Autodesk Inventor part; units mm, degrees
ref_plane "YZ Plane" through (0, 0, 0) normal (1, 0, 0) x (0, 1, 0)
ref_plane "XZ Plane" through (0, 0, 0) normal (0, 1, 0) x (-1, 0, 0)
ref_plane "XY Plane" through (0, 0, 0) normal (0, 0, 1) x (1, 0, 0)
sketch "Sketch1" plane through (0, 0, 0) normal (0, 1, 0) x (-1, 0, 0)
  line L0 (-4, 0) -> (-2, 3.4641)
  line L1 (-2, 3.4641) -> (2, 3.4641)
  line L2 (2, 3.4641) -> (4, 0)
  line L3 (4, 0) -> (2, -3.4641)
  line L4 (2, -3.4641) -> (-2, -3.4641)
  line L5 (-2, -3.4641) -> (-4, 0)
  point P0 (0, 0)
  point P1 (0, 0)
  dimension "d1" = 8
extrude "Extrusion1" add sketch "Sketch1" along normal blind 3
sketch "Sketch2" plane through (0, 0, 0) normal (0, -1, 0) x (1, 0, 0)
  circle A0 centre (0, 0) radius 3
  dimension "d4" = 6
extrude "Extrusion2" add sketch "Sketch2" along normal blind 1
sketch "Sketch3" plane through (0, -1, 0) normal (0, -1, 0) x (1, 0, 0)
  circle A0 centre (0, 0) radius 3
  circle A1 centre (0, 0) radius 3
extrude "Extrusion3" add sketch "Sketch3" along normal blind 4.5
thread "Thread1"
sketch "Sketch4" plane through (0, 3, 0) normal (0, 1, 0) x (1, 0, 0)
  point P0 (0, 0)
hole "Hole1" at (0, 3, 0) direction (0, -1, 0) diameter 3 end through all
properties material "Brass, Soft Yellow, Welded"
Input: part model. Units: mm. Frame: model coordinates. A direction names the side the tool comes from. Coordinates: 2 decimals unless noted, no trailing zeros. Loops run counter-clockwise (first coordinate to the right, second up) from the corner with the lowest first, then second, coordinate; pieces in that order, holes last.
(1) First-contact query: pin 1 Ø2 at (y, z) = (-0.5, -0.5) entering from +X; pin 2 Ø1.5 at (x, y) = (3, -2) entering from -Z; pin 3 Ø2 at (y, z) = (-2, 2.5) entering from -X; pin 4 Ø1 at (x, y) = (-1.5, -4.5) entering from +Z. Flat tips, straight axial feed; report the tip coordinate or a pass-through.
(2) Set-up query: faces 5 (the face through (2.986, 1.479, -1.756)), 6 (the face through (-3, -3, 0)). Return all of +Z, -Z, +X, -X, +Y, -Y with unobstructed straight access to the full face (end or side cutting, diameter ignored); none if empty.
(3) Section B-B on y = 2.5. Return the cut outline in (x, z), then the cut area to 3 significant figures.
(4) Material intervals for probe 1 along Z at (x, y) = (0, -1); probe 2 along Z at (x, y) = (0, 0.75); probe 3 along Y at (x, z) = (-3, -1), sorted ascending.
(5) Section A-A on x = 0. Return the cut outline in (y, z), then the cut area to 3 significant figures.
(6) Section D-D on z = 2.75. Return the cut outline in (x, y).
(7) Pull-direction query (X, two-part tool) for faces 1 (the face through (-0.07, -1.31, -1.5)), 2 (the face through (-3.014, 1.479, -1.708)), 3 (the face through (3.014, 1.479, 1.708)), 4 (the face through (0, 3, 2)); classes: released by +X, released by -X, zero draft, split by the parting line, or undercut.
(8) Section C-C on z = -0.75. Return the cut outline in (x, y), then the cut area to 3 significant figures.
Data:
1. pin 1: stops at x = 4
1. pin 2: stops at z = -1.98
1. pin 3: stops at x = -2.6
1. pin 4: stops at z = 2.83
2. face 5: -Z, +X, +Y, -Y
2. face 6: -Y
3. outline: (-4, 0) - (-2, -3.46) - (2, -3.46) - (4, 0) - (2, 3.46) - (-2, 3.46) - close; hole circle Ø3 at (0, 0)
3. area: 34.5 mm2
4. probe 1: z = -3 to -1.5, 1.5 to 3
4. probe 2: z = -3.46 to -1.5, 1.5 to 3.46
4. probe 3: y = 0 to 3
5. outline: (-5.5, -3) - (0, -3) - (0, -3.46) - (3, -3.46) - (3, -1.5) - (-5.5, -1.5) - close; (-5.5, 1.5) - (3, 1.5) - (3, 3.46) - (0, 3.46) - (0, 3) - (-5.5, 3) - close
5. area: 28.3 mm2
6. outline: (-2.41, 0) - (-1.2, 0) - (-1.2, -5.5) - (1.2, -5.5) - (1.2, 0) - (2.41, 0) - (2.41, 3) - (-2.41, 3) - close
7. face 1: undercut
7. face 2: released by -X
7. face 3: released by +X
7. face 4: zero draft
8. outline: (-3.57, 0) - (-2.9, 0) - (-2.9, -5.5) - (-1.3, -5.5) - (-1.3, 3) - (-3.57, 3) - close; (1.3, -5.5) - (2.9, -5.5) - (2.9, 0) - (3.57, 0) - (3.57, 3) - (1.3, 3) - close
8. area: 31.3 mm2
